from build123d import *

# Parameters (mm, degrees)
CROQUIS1_R              = 37.5
SALIENTE_EXTRUIR1_DEPTH = 3
CROQUIS2_R              = 32.482230575
CROQUIS2_R_2            = 29.959502021
CROQUIS2_R_3            = 24.997270629
CROQUIS2_R_4            = 22.495570161
CROQUIS2_R_5            = 17.467972247
CROQUIS2_R_6            = 14.95820612
CORTAR_EXTRUIR1_DEPTH   = 1
CROQUIS3_R              = 0.976738779
CROQUIS3_R_2            = 0.973277505
CROQUIS3_R_3            = 1.026895089
CORTAR_EXTRUIR2_DEPTH   = 3


with BuildPart() as part:
    # Croquis1 → Saliente-Extruir1 (new body)
    with BuildSketch(Plane(origin=(0, 0, 0), x_dir=(0, 0, -1), z_dir=(1, 0, 0))):
        Circle(CROQUIS1_R)
    extrude(amount=SALIENTE_EXTRUIR1_DEPTH)

    # Croquis2 → Cortar-Extruir1 (cut)
    # profile 1 of 3: a face of its own
    with BuildSketch(Plane.ZY):
        Circle(CROQUIS2_R)
        Circle(CROQUIS2_R_2, mode=Mode.SUBTRACT)
    # profile 2 of 3: a face of its own
    with BuildSketch(Plane.ZY):
        Circle(CROQUIS2_R_3)
        Circle(CROQUIS2_R_4, mode=Mode.SUBTRACT)
    # profile 3 of 3: a face of its own
    with BuildSketch(Plane.ZY):
        Circle(CROQUIS2_R_5)
        Circle(CROQUIS2_R_6, mode=Mode.SUBTRACT)
    extrude(amount=-CORTAR_EXTRUIR1_DEPTH, mode=Mode.SUBTRACT)

    # Croquis3 → Cortar-Extruir2 (cut)
    with BuildSketch(Plane.ZY):
        with Locations((16.101684192, 0)):
            Circle(CROQUIS3_R)
        with Locations((23.768998706, 0)):
            Circle(CROQUIS3_R_2)
        with Locations((31.1682253, 0)):
            Circle(CROQUIS3_R_3)
    extrude(amount=-CORTAR_EXTRUIR2_DEPTH, mode=Mode.SUBTRACT)


solid = part.part
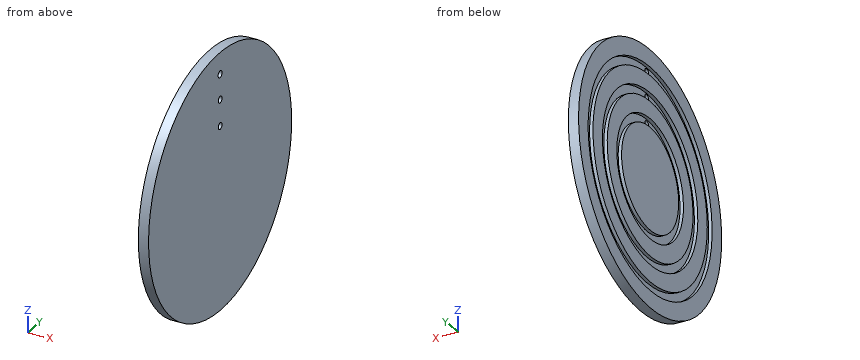
Read the model definition and answer for the solid it produces. Units are mm, in the model's axes. Coordinates: 2 decimals unless noted, no trailing zeros. Write each loop counter-clockwise with the first axis right and the second up, starting at its lowest first coordinate (ties: lowest second). Pieces come first, ordered by that corner, then holes. Notation, with made-up numbers: (-30.5, 89.25) -> (-19.5, 89.25) arc R15 cw to (-19.5, 112.25) -> close; hole circle Ø9 at (-33.5, 3.25). An arc over 180 degrees is marked (long way). Return JSON: item names as keys, results as strings.
(1) The part is cut by section C-C on x = 2.2. Give the vertices of the cut face in (y, z), then the cut area to 3 significant figures.
Answers below:
{"outline": "circle Ø75 at (0, 0); hole circle Ø2.05 at (0, 31.17); hole circle Ø1.95 at (0, 16.1); hole circle Ø1.95 at (0, 23.77)", "area": "4,410 mm^2"}
(2) The part is cut by section B-B on y = -2. Give the vertices of the cut face in (x, z).
Answers below:
{"outline": "(0, -37.45) -> (3, -37.45) -> (3, 37.45) -> (0, 37.45) -> (0, 32.42) -> (1, 32.42) -> (1, 29.89) -> (0, 29.89) -> (0, 24.92) -> (1, 24.92) -> (1, 22.41) -> (0, 22.41) -> (0, 17.35) -> (1, 17.35) -> (1, 14.82) -> (0, 14.82) -> (0, -14.82) -> (1, -14.82) -> (1, -17.35) -> (0, -17.35) -> (0, -22.41) -> (1, -22.41) -> (1, -24.92) -> (0, -24.92) -> (0, -29.89) -> (1, -29.89) -> (1, -32.42) -> (0, -32.42) -> close"}
(3) The part is cut by section D-D on y = -28. Give the vertices of the cut face in (x, z).
Answers below:
{"outline": "(0, -24.94) -> (3, -24.94) -> (3, 24.94) -> (0, 24.94) -> (0, 16.46) -> (1, 16.46) -> (1, 10.66) -> (0, 10.66) -> (0, -10.66) -> (1, -10.66) -> (1, -16.46) -> (0, -16.46) -> close"}
(4) The part is cut by section A-A on z = 0. Give the vertices of the cut face in (x, y), then the cut area to 3 significant figures.
Answers below:
{"outline": "(0, -37.5) -> (3, -37.5) -> (3, 37.5) -> (0, 37.5) -> (0, 32.48) -> (1, 32.48) -> (1, 29.96) -> (0, 29.96) -> (0, 25) -> (1, 25) -> (1, 22.5) -> (0, 22.5) -> (0, 17.47) -> (1, 17.47) -> (1, 14.96) -> (0, 14.96) -> (0, -14.96) -> (1, -14.96) -> (1, -17.47) -> (0, -17.47) -> (0, -22.5) -> (1, -22.5) -> (1, -25) -> (0, -25) -> (0, -29.96) -> (1, -29.96) -> (1, -32.48) -> (0, -32.48) -> close", "area": "210 mm^2"}
(5) Each of these flat-tipped pins is pushed along its axis until it touches: P1, Ø1.6, axis at y = 0, z = 31.17, coming from the +X side; P2, Ø1, axis at x = 2.5, y = -26, coming from the +Z side; P3, Ø1.5, axis at x = 0.5, y = -25.5, coming from the -Z side. Where does it stop, or does it pass through?
Answers below:
{"P1": "through", "P2": "z = 27.5", "P3": "z = -28.17"}
(6) Consider line 1 along Z through (x, y) = (0.5, -26); line 2 along Y through (x, z) = (0.65, 15); line 3 along X through (y, z) = (22, -11.5). Determine where each line is inside the solid, lowest interval first. Write a range as from..to.
Answers below:
{"line 1": "-27.02..-19.47, -14.89..14.89, 19.47..27.02", "line 2": "-34.37..-28.81, -25.93..-20, -16.76..-8.95, 8.95..16.76, 20..25.93, 28.81..34.37", "line 3": "1..3"}
